from build123d import *

# Parameters (mm, degrees)
M3X0_5_TAPPED_HOLE1_D     = 2.5
M3X0_5_TAPPED_HOLE1_DEPTH = 4.5
M3X0_5_TAPPED_HOLE1_TIP   = 0.751075774


with BuildPart() as part:
    # Sketch1 → Revolve1 (revolve)
    with BuildSketch(Plane.XY, mode=Mode.PRIVATE) as revolve1_sk:
        with BuildLine():
            Line((-2.5, 0), (-15, 0))
            ThreePointArc((-15, 0), (-19.069705149, 1.583048928), (-21, 5.5))
            Line((-21, 5.5), (-16, 5.5))
            Line((-16, 5.5), (-16, 13.5))
            Line((-16, 13.5), (-5, 13.5))
            Line((-5, 13.5), (-5, 5.5))
            Line((-5, 5.5), (-2.5, 3))
            Line((-2.5, 3), (-2.5, 0))
        make_face()
    revolve(revolve1_sk.sketch.rotate(Axis((0, 0, 0), (0, 1, 0)), 270), axis=Axis((0, 0, 0), (0, 1, 0)))

    # M3x0.5 Tapped Hole1
    with Locations(Plane(origin=(0, 0, 0), x_dir=(-1, 0, 0), z_dir=(0, -1, 0))):
        with Locations((12.5, 0), (0, 9.5), (-12.5, 0), (0, -9.5)):
            Hole(M3X0_5_TAPPED_HOLE1_D / 2, depth=M3X0_5_TAPPED_HOLE1_DEPTH)
            with Locations((0, 0, -(M3X0_5_TAPPED_HOLE1_DEPTH + M3X0_5_TAPPED_HOLE1_TIP / 2))):  # 118° drill point
                Cone(0, M3X0_5_TAPPED_HOLE1_D / 2, M3X0_5_TAPPED_HOLE1_TIP, mode=Mode.SUBTRACT)


solid = part.part
The model under review builds one solid part; all positions refer to its coordinate system, in mm. A direction names the side the tool comes from. Give positions to 0.01 mm unless a question says otherwise; leave off trailing zeros. Order: outer loops, then holes, each group sorted by start corner. A loop starts at its lowest first (then second) coordinate and runs counter-clockwise, first axis right, second up. Notation, with made-up numbers: M -22.5,50.5 L 10.5,50.5 A15 cw 10.5,75.5 Z; hole C 51,-11 d8. An arc over 180 degrees is marked long. Answer in a Markdown table with one row per item. Add a question column.
1. Machinability: for faces 1 (the flat face through (-4, 13.5, 4)), 2 (the cylindrical face through (-13.75, 2.28, -0.05)), 3 (the flat face through (15.5, 5.5, 4.8)), which of the approach directions +Z, -Z, +X, -X, +Y, -Y give a long, thin tool a straight path to every point of the face, cutting with its end or side? Answer none if there is none.
2. For pin 1 Ø2 at (x, y) = (-4, 3) entering from -Z; pin 2 Ø5 at (y, z) = (11, -11) entering from +X; pin 3 Ø6 at (x, y) = (-11.5, 2) entering from +Z, all flat-tipped, find the tip position at first contact; note any pin that passes through.
3. Add section A-A on y = 6.5. State the section outline as (x, z) points, plus the area to 3 significant figures.
4. To check wall thickness, follow line 1 along X through (y, z) = (4.25, 0.5); line 2 along X through (y, z) = (2.05, 9.5); line 3 along Z through (x, y) = (13.5, 1.75). State the ranges of each line that lie inside material, in increasing order.
5. Mouldability with a two-part tool opening along X and no side actions: class faces 4 (the cylindrical face through (15.62, 9.56, 3.47)), 5 (the conical face through (1.595, 3.121, 2.08)), 6 (the flat face through (0, 0, 3)) as released by +X, released by -X, zero draft, split by the parting line, or undercut.
The answers:
| question | item | result |
|---|---|---|
| 1 | face 1 | +Z, -Z, +X, -X, +Y |
| 1 | face 2 | -Y |
| 1 | face 3 | +Y |
| 2 | pin 1 | z = -20.33 |
| 2 | pin 2 | x = 13.56 |
| 2 | pin 3 | z = 18.48 |
| 3 | outline | C 0,0 d32; hole C 0,0 d10 |
| 3 | area | 726 mm2 |
| 4 | line 1 | -20.75 to -13.65, -11.35 to -3.72, 3.72 to 11.35, 13.65 to 20.75 |
| 4 | line 2 | -17.06 to -1.25, 1.25 to 17.06 |
| 4 | line 3 | -13.72 to -0.75, 0.75 to 13.72 |
| 5 | face 4 | split by the parting line |
| 5 | face 5 | undercut |
| 5 | face 6 | zero draft |
